```python
from build123d import *

# Parameters (mm, degrees)
SKETCH1_W           = 6.2
SKETCH1_H           = 10.7
BOSS_EXTRUDE1_DEPTH = 2
SKETCH2_W           = 7.1
SKETCH2_H           = 0.25368462
BOSS_EXTRUDE2_DEPTH = 40
SKETCH3_W           = 0.2
SKETCH3_H           = 0.05
BOSS_EXTRUDE3_DEPTH = 6
CUT_EXTRUDE1_DEPTH  = 0.05


with BuildPart() as part:
    # Sketch1 → Boss-Extrude1 (new body)
    with BuildSketch(Plane(origin=(0, 0, 0), x_dir=(1, 0, 0), z_dir=(0, 1, 0))):
        Polygon((-3.6, -6.1), (-3.1, -6.1), (3.1, -6.1), (3.6, -6.1), (3.6, 6.1), (-3.6, 6.1), align=None)
        with Locations((0, -11.45)):
            Rectangle(SKETCH1_W, SKETCH1_H)
    extrude(amount=BOSS_EXTRUDE1_DEPTH)

    # Sketch2 → Boss-Extrude2 (add)
    with BuildSketch(Plane(origin=(0, 0, -6.1), x_dir=(-1, 0, 0), z_dir=(0, 0, -1))):
        with Locations((0, 1)):
            Rectangle(SKETCH2_W, SKETCH2_H)
    extrude(amount=BOSS_EXTRUDE2_DEPTH)

    # Sketch3 → Boss-Extrude3 (add)
    with BuildSketch(Plane.XY.offset(16.8)):
        with Locations((0, 1)):
            Rectangle(SKETCH3_W, SKETCH3_H)
    extrude(amount=BOSS_EXTRUDE3_DEPTH)

    # Sketch4 → Cut-Extrude1 (cut)
    with BuildSketch(Plane.XZ.offset(-0.975)):
        Polygon((0.1, 22.8), (0, 22.8), (0.1, 22.5), align=None)
        Polygon((-0.1, 22.8), (-0.1, 22.5), (0, 22.8), align=None)
    extrude(amount=-CUT_EXTRUDE1_DEPTH, mode=Mode.SUBTRACT)


solid = part.part
```
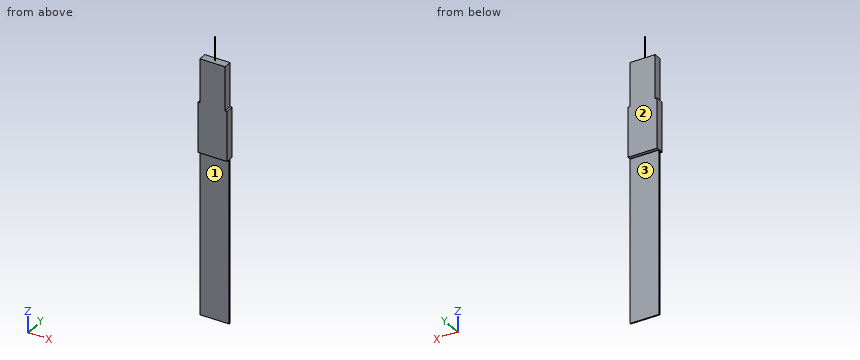
Could you check a few things on this model? Use its own coordinates, in mm. Face numbers are marked on the shaded views. A direction names the side the tool comes from. Give positions to 0.01 mm unless a question says otherwise; leave off trailing zeros. Write each loop counter-clockwise with the first axis right and the second up, starting at its lowest first coordinate (ties: lowest second). Pieces come first, ordered by that corner, then holes. Notation, with made-up numbers: (76, 33) - (103, 33) arc R17 cw to (103, 43) - close; hole circle Ø11 at (38.25, 76). An arc over 180 degrees is marked (long way). One line per item, written item: value. Start each with the question number.
Item 1: Imagine slicing it at A-A, the plane x = -2.5. List the corners of the cut face in (y, z) for me, and give its area (3 significant figures).
Item 2: Please list where these lines run through material, in increasing order: line 1 (Z direction, x = -0.5, y = 1.85); line 2 (Z direction, x = 1.5, y = 1.05); line 3 (Y direction, x = 3, z = -39.5). Write a range as from..to.
Item 3: Which directions (+Z, -Z, +X, -X, +Y, -Y) give clear straight access to the entire face, cutting with the end or side of a thin tool? Please do the marked faces 1, 2 and 3.
Item 4: Imagine slicing it at C-C, the plane z = -38.5. List the corners of the cut face in (x, y) for me.
Item 5: Imagine slicing it at B-B, the plane z = 18.5. List the corners of the cut face in (x, y) for me (3 decimals).
Item 6: I'm going to push flat-ended pins straight in: pin 1 (2 mm diameter, centred on x = 1.5, z = -25, fed in from -Y); pin 2 (1 mm diameter, centred on x = 2, z = -31.5, fed in from +Y); pin 3 (0.6 mm diameter, centred on x = -0.5, y = 1, fed in from +Z). Where does each tip first touch, or does it pass through?
Geometry says:
1. outline: (0, -6.1) - (0.87, -6.1) - (0.87, -46.1) - (1.13, -46.1) - (1.13, -6.1) - (2, -6.1) - (2, 16.8) - (0, 16.8) - close
1. area: 55.9 mm^2
2. line 1: -6.1..16.8
2. line 2: -46.1..16.8
2. line 3: 0.87..1.13
3. face 1: -Z, +X, -X, -Y
3. face 2: +Z, -Z, +X, -X, +Y
3. face 3: -Z, +X, -X, +Y
4. outline: (-3.55, 0.87) - (3.55, 0.87) - (3.55, 1.13) - (-3.55, 1.13) - close
5. outline: (-0.1, 0.975) - (0.1, 0.975) - (0.1, 1.025) - (-0.1, 1.025) - close
6. pin 1: y = 0.87
6. pin 2: y = 1.13
6. pin 3: z = 16.8
